from build123d import *

# Parameters (mm, degrees)
SKETCH_1_R      = 2
EXTRUDE_1_DEPTH = 3
FILLET_1_R      = 5


with BuildPart() as part:
    # 草图1 → 凸台-拉伸1 (new body)
    with BuildSketch(Plane.XY):
        with BuildLine():
            Line((-15, 9.366750419), (-15, -30.633249581))
            Line((-15, -30.633249581), (15, -30.633249581))
            Line((15, -30.633249581), (15, 9.366750419))
            ThreePointArc((15, 9.366750419), (0, 24.366750419), (-15, 9.366750419))
        make_face()
        with Locations((-7.5, -9.633249581)):
            Circle(SKETCH_1_R, mode=Mode.SUBTRACT)
        with Locations((-7.5, -23.633249581)):
            Circle(SKETCH_1_R, mode=Mode.SUBTRACT)
        with Locations(Location((7.5, -23.633249581, 0), (0, 0, 180))):
            Circle(SKETCH_1_R, mode=Mode.SUBTRACT)
        with Locations(Location((7.5, -9.633249581, 0), (0, 0, 180))):
            Circle(SKETCH_1_R, mode=Mode.SUBTRACT)
        with BuildLine():
            Line((3, 5.366750419), (-3, 5.366750419))
            ThreePointArc((-3, 5.366750419), (0, 14.366750419), (3, 5.366750419))
        make_face(mode=Mode.SUBTRACT)
    extrude(amount=EXTRUDE_1_DEPTH)

    # 圆角1
    fillet_1_edges = [part.edges().sort_by_distance(p)[0] for p in [
        (15, -30.633249581, 1.5),
        (-15, -30.633249581, 1.5),
    ]]
    fillet(fillet_1_edges, radius=FILLET_1_R)


solid = part.part
Model file for the job. Use its own axes, mm. A direction names the side the tool comes from. Give positions to 0.01 mm unless a question says otherwise; leave off trailing zeros. Order: outer loops, then holes, each group sorted by start corner. A loop starts at its lowest first (then second) coordinate and runs counter-clockwise, first axis right, second up. Notation, with made-up numbers: M 7.25,28 L 25.25,28 A23 ccw 25.25,43 Z; hole C -24,34.25 d8. An arc over 180 degrees is marked long. Write item = value, one per line.
Q1. Cut at B-B, the plane z = 1.25. List the corners of the cut face in (x, y), then the cut area to 3 significant figures.
Derived:
outline = M -15,-25.63 A5 ccw -10,-30.63 L 10,-30.63 A5 ccw 15,-25.63 L 15,9.37 A15 ccw -15,9.37 Z; hole C -7.5,-23.63 d4; hole C -7.5,-9.63 d4; hole M -3,5.37 L 3,5.37 A5 ccw long Z; hole C 7.5,-23.63 d4; hole C 7.5,-9.63 d4
area = 1,420 mm2
Q2. Cut at C-C, the plane x = -7.5. List the corners of the cut face in (y, z), then the cut area to 3 significant figures.
Derived:
outline = M -30.63,0 L -25.63,0 L -25.63,3 L -30.63,3 Z; M -21.63,0 L -11.63,0 L -11.63,3 L -21.63,3 Z; M -7.63,0 L 22.36,0 L 22.36,3 L -7.63,3 Z
area = 135 mm2
Q3. Tool access for faces 1 (the flat face through (-15, -8, 1)), 2 (the flat face through (0, 5.367, 1)): list every direction of +Z, -Z, +X, -X, +Y, -Y with a clear straight run to the whole face (end or side of a thin tool).
Derived:
face_1 = +Z, -Z, -X, +Y, -Y
face_2 = +Z, -Z
Q4. Drill centre lines: line 1 (Y direction, x = -6, z = 1); line 2 (Y direction, x = 0, z = 1.35); line 3 (Y direction, x = -4.5, z = 1.7). Where is each one in solid material? Low to high. Write a range as [from, to].
Derived:
line_1 = [-30.63, -24.96], [-22.31, -10.96], [-8.31, 23.11]
line_2 = [-30.63, 5.37], [14.37, 24.37]
line_3 = [-30.63, 7.19], [11.55, 23.68]
Q5. Cut at A-A, the plane x = 0. List the corners of the cut face in (y, z), then the cut area to 3 significant figures.
Derived:
outline = M -30.63,0 L 5.37,0 L 5.37,3 L -30.63,3 Z; M 14.37,0 L 24.37,0 L 24.37,3 L 14.37,3 Z
area = 138 mm2
Q6. Two-plate mould, pull along X, no slides. Class faces 3 (the flat face through (0, -3, 0)), 4 (the cylindrical face through (7.76, -25.616, 1.479)), 5 (the cylindrical face through (-9.087, -24.85, 1.479)), 6 (the cylindrical face through (0.33, 24.363, 1.479)): pulls with the +X half, pulls with the -X half, needs draft (parallel to the pull), parting line crosses it, or undercut.
Derived:
face_3 = needs draft
face_4 = undercut
face_5 = undercut
face_6 = parting line crosses it
Q7. Flat gauge pins, fed straight in: pin 1 (4.5 mm diameter, centred on x = -7.5, y = -23.63, fed in from -Z); pin 2 (3 mm diameter, centred on x = 7.5, y = -9.63, fed in from +Z). Where does each tip first touch, or does it go through?
Derived:
pin_1 = 0
pin_2 = through
Q8. Cut at D-D, the plane y = 16. List the corners of the cut face in (x, z), then the cut area to 3 significant figures.
Derived:
outline = M -13.45,0 L 13.45,0 L 13.45,3 L -13.45,3 Z
area = 80.7 mm2
